Autodesk Fusion 360 part; units mm, degrees
sketch "Sketch1" plane through (0, 0, 0) normal (0, 0, 1) x (1, 0, 0) in component "5S100ABMS"
  line L0 (-30.4, 21.15) -> (30.4, 21.15)
  line L1 (30.4, 21.15) -> (30.4, -21.15)
  line L2 (30.4, -21.15) -> (-30.4, -21.15)
  line L3 (-30.4, -21.15) -> (-30.4, 21.15)
  line L4 (-30.4, 21.15) -> (30.4, -21.15) construction
  line L5 (30.4, 21.15) -> (-30.4, -21.15) construction
  line L6 (30.4, 21.15) -> (27.1, 21.15) construction
  line L7 (27.1, 21.15) -> (27.1, 18.45) construction
  line L8 (27.1, 18.45) -> (30.4, 18.45) construction
  line L9 (30.4, 18.45) -> (30.4, 21.15) construction
  line L10 (-30.4, -19.35) -> (-27.9, -19.35) construction
  line L11 (-27.9, -19.35) -> (-27.9, -21.15) construction
  line L12 (-27.9, -21.15) -> (-30.4, -21.15) construction
  line L13 (-30.4, -21.15) -> (-30.4, -19.35) construction
  circle A0 centre (25.3, 16.65) radius 1.8
  circle A1 centre (-26.3, -17.75) radius 1.6
  line L14 (25.3, 16.65) -> (27.1, 16.65) construction
  line L15 (27.1, 16.65) -> (27.1, 18.45) construction
  line L16 (27.1, 18.45) -> (25.3, 18.45) construction
  line L17 (25.3, 18.45) -> (25.3, 16.65) construction
  line L18 (-26.3, -17.75) -> (-27.9, -17.75) construction
  line L19 (-27.9, -17.75) -> (-27.9, -19.35) construction
  line L20 (-27.9, -19.35) -> (-26.3, -19.35) construction
  line L21 (-26.3, -19.35) -> (-26.3, -17.75) construction
  dimension "Length" = 60.8
  dimension "Width" = 42.3
  dimension "d3" = 3.3
  dimension "d4" = 2.7
  dimension "d5" = 2.5
  dimension "d6" = 1.8
  dimension "d7" = 3.6
  dimension "d8" = 3.2
extrude "Extrude1" add sketch "Sketch1" along normal blind 1.6 in component "5S100ABMS"
sketch "Sketch2" plane through (0, 0, 1.6) normal (0, 0, 1) x (1, 0, 0) in component "5S100ABMS"
  circle A0 centre (-26.3, -17.75) radius 1.6
  circle A1 centre (25.3, 16.65) radius 1.8
  line L0 (-30.4, -21.15) -> (30.4, -21.15)
  line L1 (30.4, -21.15) -> (30.4, 21.15)
  line L2 (30.4, 21.15) -> (-30.4, 21.15)
  line L3 (-30.4, 21.15) -> (-30.4, -21.15)
  line L4 (-29.4367, -6.6251) -> (-29.4367, -0.6251)
  line L5 (-23.4367, -0.6251) -> (-23.4367, -6.6251)
  line L6 (-29.4367, -0.6251) -> (-23.4367, -0.6251)
  line L7 (-29.4367, -6.6251) -> (-23.4367, -0.6251) construction
  line L8 (-23.4367, -6.6251) -> (-29.4367, -6.6251)
  line L9 (-23.4367, -6.6251) -> (-29.4367, -0.6251) construction
  line L10 (-22.2878, -15.0909) -> (-22.2878, -9.0909)
  line L11 (-16.2878, -9.0909) -> (-16.2878, -15.0909)
  line L12 (-22.2878, -9.0909) -> (-16.2878, -9.0909)
  line L13 (-22.2878, -15.0909) -> (-16.2878, -9.0909) construction
  line L14 (-16.2878, -15.0909) -> (-22.2878, -15.0909)
  line L15 (-16.2878, -15.0909) -> (-22.2878, -9.0909) construction
  line L16 (-14.6686, -15.0909) -> (-14.6686, -9.0909)
  line L17 (-8.6686, -9.0909) -> (-8.6686, -15.0909)
  line L18 (-14.6686, -9.0909) -> (-8.6686, -9.0909)
  line L19 (-14.6686, -15.0909) -> (-8.6686, -9.0909) construction
  line L20 (-8.6686, -15.0909) -> (-14.6686, -15.0909)
  line L21 (-8.6686, -15.0909) -> (-14.6686, -9.0909) construction
  line L22 (-7.1435, -15.0909) -> (-7.1435, -9.0909)
  line L23 (-1.1435, -9.0909) -> (-1.1435, -15.0909)
  line L24 (-7.1435, -9.0909) -> (-1.1435, -9.0909)
  line L25 (-7.1435, -15.0909) -> (-1.1435, -9.0909) construction
  line L26 (-1.1435, -15.0909) -> (-7.1435, -15.0909)
  line L27 (-1.1435, -15.0909) -> (-7.1435, -9.0909) construction
  line L28 (0.3817, -15.0909) -> (0.3817, -9.0909)
  line L29 (6.3817, -9.0909) -> (6.3817, -15.0909)
  line L30 (0.3817, -9.0909) -> (6.3817, -9.0909)
  line L31 (0.3817, -15.0909) -> (6.3817, -9.0909) construction
  line L32 (6.3817, -15.0909) -> (0.3817, -15.0909)
  line L33 (6.3817, -15.0909) -> (0.3817, -9.0909) construction
  line L34 (7.9839, -15.0909) -> (7.9839, -9.0909)
  line L35 (13.9839, -9.0909) -> (13.9839, -15.0909)
  line L36 (7.9839, -9.0909) -> (13.9839, -9.0909)
  line L37 (7.9839, -15.0909) -> (13.9839, -9.0909) construction
  line L38 (13.9839, -15.0909) -> (7.9839, -15.0909)
  line L39 (13.9839, -15.0909) -> (7.9839, -9.0909) construction
  line L40 (15.5731, -15.0909) -> (15.5731, -9.0909)
  line L41 (21.5731, -9.0909) -> (21.5731, -15.0909)
  line L42 (15.5731, -9.0909) -> (21.5731, -9.0909)
  line L43 (15.5731, -15.0909) -> (21.5731, -9.0909) construction
  line L44 (21.5731, -15.0909) -> (15.5731, -15.0909)
  line L45 (21.5731, -15.0909) -> (15.5731, -9.0909) construction
  line L46 (22.9058, -15.0909) -> (22.9058, -9.0909)
  line L47 (28.9058, -9.0909) -> (28.9058, -15.0909)
  line L48 (22.9058, -9.0909) -> (28.9058, -9.0909)
  line L49 (22.9058, -15.0909) -> (28.9058, -9.0909) construction
  line L50 (28.9058, -15.0909) -> (22.9058, -15.0909)
  line L51 (28.9058, -15.0909) -> (22.9058, -9.0909) construction
  line L52 (-16.3819, -6.6251) -> (-22.3819, -6.6251)
  line L53 (-1.2375, -6.6251) -> (-7.2375, -0.6251) construction
  line L54 (0.2876, -6.6251) -> (0.2876, -0.6251)
  line L55 (-1.2375, -0.6251) -> (-1.2375, -6.6251)
  line L56 (7.9089, -6.6251) -> (7.9089, -0.6251)
  line L57 (13.9089, -6.6251) -> (7.9089, -0.6251) construction
  line L58 (-22.3819, -6.6251) -> (-16.3819, -0.6251) construction
  line L59 (-16.3819, -6.6251) -> (-22.3819, -0.6251) construction
  line L60 (28.8058, -6.6251) -> (22.8058, -6.6251)
  line L61 (6.2876, -0.6251) -> (6.2876, -6.6251)
  line L62 (-14.7627, -6.6251) -> (-14.7627, -0.6251)
  line L63 (15.479, -6.6251) -> (21.479, -0.6251) construction
  line L64 (-1.2375, -6.6251) -> (-7.2375, -6.6251)
  line L65 (-14.7627, -6.6251) -> (-8.7627, -0.6251) construction
  line L66 (22.8058, -6.6251) -> (22.8058, -0.6251)
  line L67 (-7.2375, -6.6251) -> (-7.2375, -0.6251)
  line L68 (7.9089, -0.6251) -> (13.9089, -0.6251)
  line L69 (22.8058, -6.6251) -> (28.8058, -0.6251) construction
  line L70 (21.479, -6.6251) -> (15.479, -0.6251) construction
  line L71 (28.8058, -0.6251) -> (28.8058, -6.6251)
  line L72 (0.2876, -0.6251) -> (6.2876, -0.6251)
  line L73 (-22.3819, -0.6251) -> (-16.3819, -0.6251)
  line L74 (13.9089, -0.6251) -> (13.9089, -6.6251)
  line L75 (-8.7627, -0.6251) -> (-8.7627, -6.6251)
  line L76 (-16.3819, -0.6251) -> (-16.3819, -6.6251)
  line L77 (22.8058, -0.6251) -> (28.8058, -0.6251)
  line L78 (21.479, -0.6251) -> (21.479, -6.6251)
  line L79 (15.479, -0.6251) -> (21.479, -0.6251)
  line L80 (-7.2375, -6.6251) -> (-1.2375, -0.6251) construction
  line L81 (-8.7627, -6.6251) -> (-14.7627, -6.6251)
  line L82 (28.8058, -6.6251) -> (22.8058, -0.6251) construction
  line L83 (-14.7627, -0.6251) -> (-8.7627, -0.6251)
  line L84 (-22.3819, -6.6251) -> (-22.3819, -0.6251)
  line L85 (7.9089, -6.6251) -> (13.9089, -0.6251) construction
  line L86 (0.2876, -6.6251) -> (6.2876, -0.6251) construction
  line L87 (-7.2375, -0.6251) -> (-1.2375, -0.6251)
  line L88 (13.9089, -6.6251) -> (7.9089, -6.6251)
  line L89 (-8.7627, -6.6251) -> (-14.7627, -0.6251) construction
  line L90 (21.479, -6.6251) -> (15.479, -6.6251)
  line L91 (6.2876, -6.6251) -> (0.2876, -6.6251)
  line L92 (6.2876, -6.6251) -> (0.2876, -0.6251) construction
  line L93 (15.479, -6.6251) -> (15.479, -0.6251)
  line L94 (-24.0917, 19.3813) -> (-19.3155, 19.3813)
  line L95 (-19.3155, 19.3813) -> (-19.3155, 9.2896)
  line L96 (-19.3155, 9.2896) -> (-24.0917, 9.2896)
  line L97 (-24.0917, 9.2896) -> (-24.0917, 19.3813)
  point P0 (-26.4367, -3.6251)
  point P1 (-19.3819, -3.6251)
  point P2 (-19.2878, -12.0909)
  point P3 (-11.6686, -12.0909)
  point P4 (-4.1435, -12.0909)
  point P5 (3.3817, -12.0909)
  point P6 (10.9839, -12.0909)
  point P7 (18.5731, -12.0909)
  point P8 (25.9058, -12.0909)
  point P9 (-19.3819, -3.6251)
  point P10 (10.9089, -3.6251)
  point P11 (-11.7627, -3.6251)
  point P12 (18.479, -3.6251)
  point P13 (3.2876, -3.6251)
  point P14 (-4.2375, -3.6251)
  point P15 (25.8058, -3.6251)
  dimension "d13" = 6
  dimension "d14" = 6
  dimension "d17" = 6
  dimension "d18" = 6
  dimension "d19" = 6
  dimension "d20" = 6
  dimension "d21" = 6
  dimension "d22" = 6
  dimension "d23" = 6
  dimension "d24" = 6
  dimension "d25" = 6
  dimension "d26" = 6
  dimension "d27" = 6
  dimension "d28" = 6
  dimension "d29" = 6
  dimension "d30" = 6
  dimension "d31" = 6
  dimension "d32" = 6
  dimension "d33" = 6
  dimension "d34" = 6
  dimension "d35" = 6
  dimension "d36" = 6
  dimension "d37" = 6
  dimension "d38" = 6
  dimension "d39" = 6
  dimension "d40" = 6
  dimension "d41" = 6
  dimension "d42" = 6
  dimension "d43" = 6
  dimension "d44" = 6
  dimension "d45" = 4.7762
extrude "Extrude2" add sketch "Sketch2" along normal blind 0.94 contours L94 L95 L96 L97 in component "5S100ABMS"
extrude "Extrude3" add sketch "Sketch2" along normal blind 2.25 contours L4 L5 L6 L8 | L10 L11 L12 L14 | L16 L17 L18 L20 | L22 L23 L24 L26 | L28 L29 L30 L32 | L34 L35 L36 L38 | L40 L41 L42 L44 | L46 L47 L48 L50 | L52 L73 L76 L84 | L54 L61 L72 L91 | L55 L64 L67 L87 | L56 L68 L74 L88 | L60 L66 L71 L77 | L62 L75 L81 L83 | L78 L79 L90 L93 in component "5S100ABMS"
component "5S100ABMS" placed x (1, 0, 0) y (0, 1, 0) z (0, 0, 1) at (0, 0, 0)
equation "d46 = 2.54 mm - Thickness"
equation "d48 = 3.85 mm - Thickness"
Can you work these out from the model? Positions are in its coordinate system, mm. A direction names the side the tool comes from. Coordinates: 2 decimals unless noted, no trailing zeros. Loops run counter-clockwise (first coordinate to the right, second up) from the corner with the lowest first, then second, coordinate; pieces in that order, holes last. Notation, with made-up numbers: (-39.75, 5) - (15.25, 5) arc R19 ccw to (15.25, 11) - close; hole circle Ø11 at (53, 53.5). An arc over 180 degrees is marked (long way). Answer as CSV lines item,"result". Start each with the question number.
1) I need wall thicknesses on line 1 (Y direction, x = 25, z = 2.95); line 2 (Y direction, x = -26.3, z = 1.1); line 3 (Z direction, x = 27, y = 10). Which ranges of each line are inside material? Lowest first, please. Write a range as from..to.
2) Which directions (+Z, -Z, +X, -X, +Y, -Y) give clear straight access to the entire face, cutting with the end or side of a thin tool? Please do faces 3 (the flat face through (3, -0.625, 3)), 4 (the flat face through (3, -9.091, 3)), 5 (the flat face through (-1.144, -12, 3)).
3) Thinking about a two-plate mould opening in X: for faces 1 (the flat face through (-12, -15.091, 3)), 2 (the cylindrical face through (-26.508, -19.336, 0.789)), which applies, pulls with the +X half, pulls with the -X half, needs draft (parallel to the pull), parting line crosses it, or undercut?
4) Suppose I cut it at A-A (y = -17.75). Please give me the cut outline in (x, z).
5) For pin 1 (1.1 mm diameter, centred on x = 25.5, z = 2.5, fed in from -Y); pin 2 (0.7 mm diameter, centred on y = -11.5, z = 3, fed in from +X); pin 3 (1.8 mm diameter, centred on x = -3.5, z = 3.5, fed in from +Y), each with a flat end and sliding along its axis, tell me the tip position at first contact or that it passes through.
6) Suppose I cut it at B-B (x = 25.3). Please give me the cut outline in (y, z), plus the area to 3 significant figures.
7) Suppose I cut it at D-D (x = -11.5). Please give me the cut outline in (y, z).
Check result:
1,line 1,"y = -15.09..-9.09, -6.63..-0.63"
1,line 2,"y = -21.15..-19.35, -16.15..21.15"
1,line 3,"z = 0..1.6"
2,face 3,"+Z, +X, -X, +Y"
2,face 4,"+Z, +X, -X"
2,face 5,"+Z, +Y, -Y"
3,face 1,"needs draft"
3,face 2,"undercut"
4,outline,"(-30.4, 0) - (-27.9, 0) - (-27.9, 1.6) - (-30.4, 1.6) - close; (-24.7, 0) - (30.4, 0) - (30.4, 1.6) - (-24.7, 1.6) - close"
5,pin 1,"stops at y = -15.09"
5,pin 2,"stops at x = 28.91"
5,pin 3,"stops at y = -0.63"
6,outline,"(-21.15, 0) - (14.85, 0) - (14.85, 1.6) - (-0.63, 1.6) - (-0.63, 3.85) - (-6.63, 3.85) - (-6.63, 1.6) - (-9.09, 1.6) - (-9.09, 3.85) - (-15.09, 3.85) - (-15.09, 1.6) - (-21.15, 1.6) - close; (18.45, 0) - (21.15, 0) - (21.15, 1.6) - (18.45, 1.6) - close"
6,area,"88.9 mm²"
7,outline,"(-21.15, 0) - (21.15, 0) - (21.15, 1.6) - (-0.63, 1.6) - (-0.63, 3.85) - (-6.63, 3.85) - (-6.63, 1.6) - (-9.09, 1.6) - (-9.09, 3.85) - (-15.09, 3.85) - (-15.09, 1.6) - (-21.15, 1.6) - close"
